The figure shows three views and two pictorial views of one solid part (mm, origin at its lowest corner). Answer the questions. A direction names the side the tool comes from. Give positions to 0.01 mm unless a question says otherwise; leave off trailing zeros. Loops run counter-clockwise (first coordinate to the right, second up) from the corner with the lowest first, then second, coordinate; pieces in that order, holes last. Notation, with made-up numbers: (8, 23) - (33, 23) arc R18 cw to (33, 57) - close; hole circle Ø10 at (8.5, -23). An arc over 180 degrees is marked (long way). Write item = value, one per line.
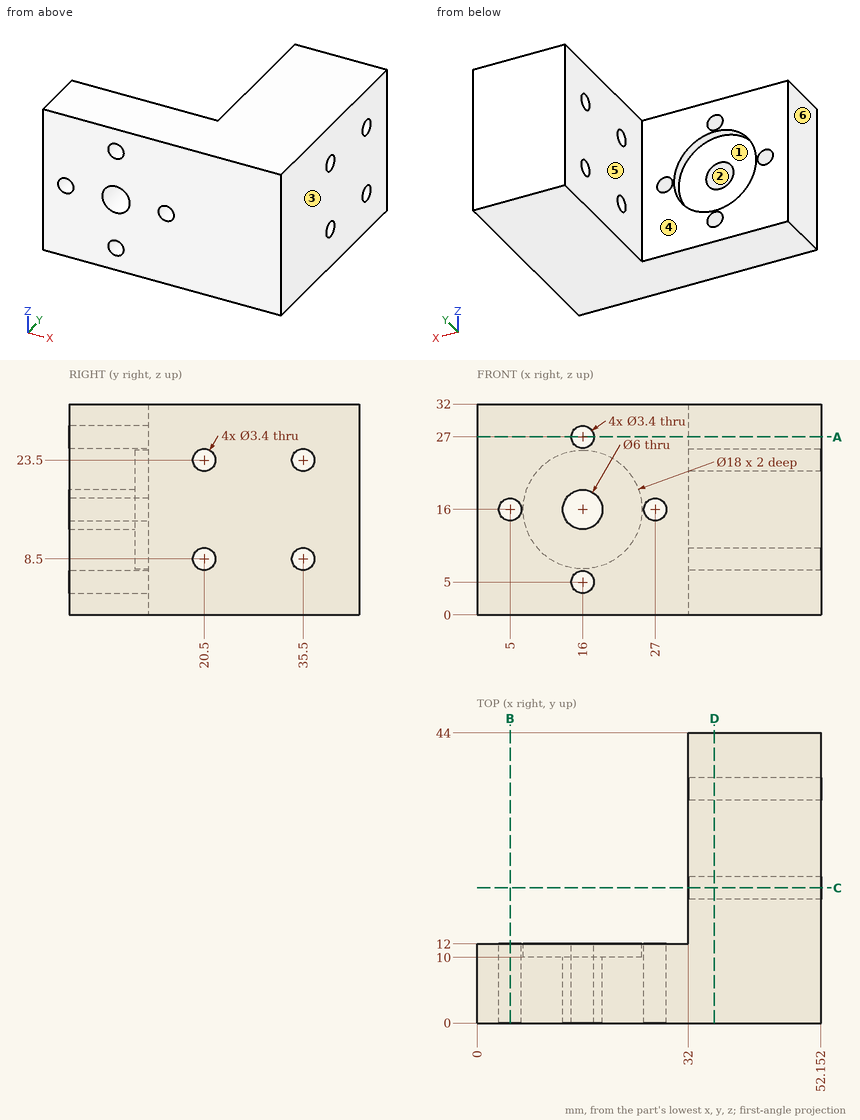
1) A cutting plane is placed at D-D on x = 36. Determine the outline of the cut face in (y, z), then the cut area to 3 significant figures.
Output:
outline = (0, 0) - (44, 0) - (44, 32) - (0, 32) - close; hole circle Ø3.4 at (20.5, 8.5); hole circle Ø3.4 at (20.5, 23.5); hole circle Ø3.4 at (35.5, 8.5); hole circle Ø3.4 at (35.5, 23.5)
area = 1,370 mm²
2) The mould has two halves that part along X. Classify the marked faces 1, 2, 3 and 4: pulls with the +X half, pulls with the -X half, needs draft (parallel to the pull), parting line crosses it, or undercut.
Output:
face_1 = undercut
face_2 = undercut
face_3 = pulls with the +X half
face_4 = needs draft
3) Each of these flat-tipped pins is pushed along its axis until it touches: P1, Ø10, axis at x = 13, z = 13, coming from the +Y side; P2, Ø3, axis at x = 5, z = 16, coming from the +Y side; P3, Ø9.5, axis at y = 28, z = 9.5, coming from the -X side; P4, Ø9, axis at x = 19.5, z = 18.5, coming from the +Y side. Where does it stop, or does it pass through?
Output:
P1 = 12
P2 = through
P3 = 32
P4 = 10
4) A cutting plane is placed at A-A on z = 27. Determine the outline of the cut face in (x, y).
Output:
outline = (0, 0) - (14.3, 0) - (14.3, 12) - (0, 12) - close; (17.7, 0) - (52.15, 0) - (52.15, 44) - (32, 44) - (32, 12) - (17.7, 12) - close
5) A tool of negligible diameter and unlimited length cuts with its end or side. For the marked faces 5 and 6, from which of +Z, -Z, +X, -X, +Y, -Y can it reach the whole face along a straight path? Write none if from no direction.
Output:
face_5 = +Z, -Z, -X, +Y
face_6 = +Z, -Z, -X, +Y, -Y
6) A cutting plane is placed at C-C on y = 20.5. Determine the outline of the cut face in (x, z), then the cut area to 3 significant figures.
Output:
outline = (32, 0) - (52.15, 0) - (52.15, 6.8) - (32, 6.8) - close; (32, 10.2) - (52.15, 10.2) - (52.15, 21.8) - (32, 21.8) - close; (32, 25.2) - (52.15, 25.2) - (52.15, 32) - (32, 32) - close
area = 508 mm²
7) A cutting plane is placed at B-B on x = 5. Determine the outline of the cut face in (y, z).
Output:
outline = (0, 0) - (12, 0) - (12, 14.3) - (0, 14.3) - close; (0, 17.7) - (12, 17.7) - (12, 32) - (0, 32) - close
8) Find the intervals of material crossed by probe 1 along X at (y, z) = (7.5, 16); probe 2 along Y at (x, z) = (40.75, 23.5); probe 3 along X at (y, z) = (17, 27), in increasing order.
Output:
probe_1 = 0 to 3.3, 6.7 to 13, 19 to 25.3, 28.7 to 52.15
probe_2 = 0 to 18.8, 22.2 to 33.8, 37.2 to 44
probe_3 = 32 to 52.15
